Read the model definition and answer for the solid it produces. Units are mm, in the model's axes. A direction names the side the tool comes from. Coordinates: 2 decimals unless noted, no trailing zeros. Write each loop counter-clockwise with the first axis right and the second up, starting at its lowest first coordinate (ties: lowest second). Pieces come first, ordered by that corner, then holes.
(1) Determine the mould class of faces 1 (the flat face through (3, 9, 0)), 2 (the cylindrical face through (8.03, 2.84, 0.37)), 3 (the flat face through (3, 0, 0)), 4 (the cylindrical face through (1.49, 4.56, 4.15)) for opening direction Y: pulls with the +Y half, pulls with the -Y half, needs draft (parallel to the pull), parting line crosses it, or undercut.
(2) The part is cut by section C-C, the plane y = 1.5. Determine the outline of the cut face in (x, z).
(3) The part is cut by section B-B, the plane z = 0. Determine the outline of the cut face in (x, y).
(4) The part is cut by section D-D, the plane y = 5. Determine the outline of the cut face in (x, z), and give its area (3 significant figures).
(5) The part is cut by section A-A, the plane x = 7.5. Determine the outline of the cut face in (y, z).
(6) Which of the six approach directions +Z, -Z, +X, -X, +Y, -Y give full straight-line access (tool end or side, diameter ignored) to faces 5 (the flat face through (0.5, 4.4, 3.65)), 6 (the cylindrical face through (-3.65, 4.44, 0.08)), 7 (the flat face through (6, 5, 0)), 8 (the flat face through (6.5, 4.4, 3.65))?
(7) Given pin 1 (0.8 mm diameter, centred on x = 0.5, y = 5, fed in from +Z), flat-ended and moving along its own axis, determine where the tip first touches the part or whether it passes through.
(8) Straight lines are drawn through the part: line 1 along Y through (x, z) = (9.1, 0); line 2 along Y through (x, z) = (8.75, 0.75); line 3 along Z through (x, y) = (2.5, 1.25). For each, find the intervals that lie inside material, in ascending order.
Autodesk Inventor part; units mm, degrees
ref_plane "YZ Plane" through (0, 0, 0) normal (1, 0, 0) x (0, 1, 0)
ref_plane "XZ Plane" through (0, 0, 0) normal (0, 1, 0) x (-1, 0, 0)
ref_plane "XY Plane" through (0, 0, 0) normal (0, 0, 1) x (1, 0, 0)
sketch "Sketch1" plane through (0, 0, 0) normal (0, 1, 0) x (-1, 0, 0)
  arc A0 (0, -3.65) -> (0, 3.65) centre (0, 0) ccw
  line L0 (0, 3.65) -> (-10, 3.65)
  line L1 (-10, 3.65) -> (-10, -3.65)
  line L2 (-10, -3.65) -> (0, -3.65)
  line L3 (0, 3.65) -> (0, -3.65)
  dimension "d0" = 10
  dimension "d1" = 7.3
extrude "Extrusion1" add sketch "Sketch1" along normal blind 9
sketch "Sketch2" plane through (0, 9, 0) normal (0, 1, 0) x (1, 0, 0)
  line L0 (9, -3.65) -> (10, -3.65)
  arc A0 (9, -3.65) -> (10, -3.65) centre (9.5, -3.65) ccw
  point P0 (0, 0)
  dimension "d4" = 1
extrude "Extrusion2" add sketch "Sketch2" against normal blind 9
pattern_linear "Rectangular Pattern1" count 5 spacing 2 along (-1, 0, 0) of "Extrusion2"
sketch "Sketch3" plane through (10, 0, -3.65) normal (1, 0, 0) x (0, 0, -1)
  line L0 (-3.65, 0) -> (-3.65, 9)
  line L1 (0, 9) -> (-7.3, 9)
  circle A0 centre (-3.65, 4.5) radius 1.7
  dimension "d10" = 3.4
extrude "Extrusion3" cut sketch "Sketch3" against normal blind 4
properties part number "XY_Tensioner" material "ABS Plastic"
Computed:
1. face 1: pulls with the +Y half
1. face 2: undercut
1. face 3: pulls with the -Y half
1. face 4: needs draft
2. outline: (0, -3.65) - (10, -3.65) - (10, 3.65) arc R0.5 ccw to (9, 3.65) - (8, 3.65) arc R0.5 ccw to (7, 3.65) - (6, 3.65) arc R0.5 ccw to (5, 3.65) - (4, 3.65) arc R0.5 ccw to (3, 3.65) - (2, 3.65) arc R0.5 ccw to (1, 3.65) - (0, 3.65) arc R3.65 ccw to start
3. outline: (-3.65, 0) - (10, 0) - (10, 2.8) - (6, 2.8) - (6, 6.2) - (10, 6.2) - (10, 9) - (-3.65, 9) - close
4. outline: (0, -3.65) - (10, -3.65) - (10, -1.62) - (6, -1.62) - (6, 1.62) - (10, 1.62) - (10, 3.65) arc R0.5 ccw to (9, 3.65) - (8, 3.65) arc R0.5 ccw to (7, 3.65) - (6, 3.65) arc R0.5 ccw to (5, 3.65) - (4, 3.65) arc R0.5 ccw to (3, 3.65) - (2, 3.65) arc R0.5 ccw to (1, 3.65) - (0, 3.65) arc R3.65 ccw to start
4. area: 82.9 mm2
5. outline: (0, -3.65) - (9, -3.65) - (9, 4.15) - (0, 4.15) - close; hole circle Ø3.4 at (4.5, 0)
6. face 5: +Z, -X, +Y, -Y
6. face 6: -X, +Y, -Y
6. face 7: +X
6. face 8: +Z, +Y, -Y
7. pin 1: stops at z = 3.65
8. line 1: y = 0 to 2.8, 6.2 to 9
8. line 2: y = 0 to 2.97, 6.03 to 9
8. line 3: z = -3.65 to 3.65
